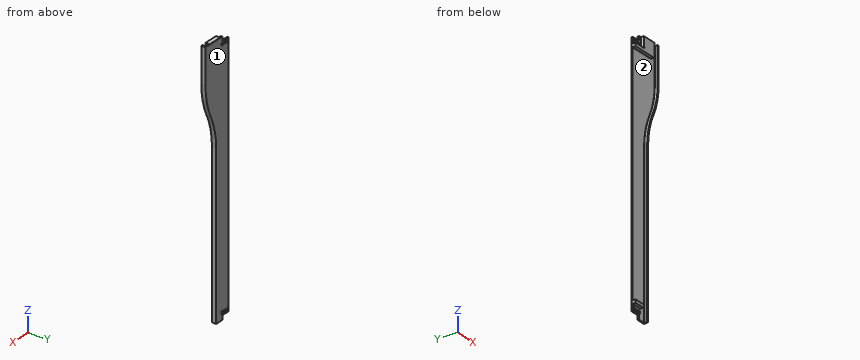
from build123d import *

# Parameters (mm, degrees)
EXTRUDE1_DEPTH                 = 10
EXTRUDE2_DEPTH                 = 7
SKETCH5_W                      = 20
SKETCH5_H                      = 15
SKETCH5_W_2                    = 26
EXTRUDE3_DEPTH                 = 7
SKETCH15_W                     = 6
SKETCH15_H                     = 10.7
SKETCH15_H_2                   = 25.7
EXTRUDE9_DEPTH                 = 7
F_8_CLEARANCE_HOLE1_AT_2_COUNT = 2
F_8_CLEARANCE_HOLE1_AT_2_PITCH = 15
EXTRUDE6_DEPTH                 = 4
SKETCH16_R                     = 1.5875
EXTRUDE10_DEPTH                = 7
CHAMFER1_SIZE                  = 0.3
CHAMFER2_SIZE                  = 0.5
CHAMFER3_SIZE                  = 0.3
FILLET3_R                      = 3
FILLET2_R                      = 0.5


with BuildPart() as part:
    # Sketch1 → Extrude1 (new body)
    with BuildSketch(Plane(origin=(0, 0, 0), x_dir=(1, 0, 0), z_dir=(0, 1, 0))):
        with BuildLine():
            Line((-93.1, 756.2), (-145.1, 756.2))
            Line((-145.1, 756.2), (-145.1, 766.9))
            Line((-145.1, 766.9), (-165.1, 766.9))
            Line((-165.1, 766.9), (-165.1, 1360.9))
            Line((-165.1, 1360.9), (-145.1, 1360.9))
            Line((-145.1, 1360.9), (-145.1, 1371.6))
            Line((-145.1, 1371.6), (-126.1, 1371.6))
            Line((-126.1, 1371.6), (-126.1, 990))
            ThreePointArc((-126.1, 990), (-121.926260039, 951.603222791), (-109.6, 915))
            ThreePointArc((-109.6, 915), (-97.273739961, 878.396777209), (-93.1, 840))
            Line((-93.1, 840), (-93.1, 756.2))
        make_face()
    extrude(amount=-EXTRUDE1_DEPTH)

    # Sketch4 → Extrude2 (cut)
    with BuildSketch(Plane.XZ.offset(10)):
        with BuildLine():
            Line((-165.1, -789.4), (-106.1, -789.4))
            Line((-106.1, -789.4), (-106.1, -756.2))
            Line((-106.1, -756.2), (-96.1, -756.2))
            Line((-96.1, -756.2), (-96.1, -840))
            ThreePointArc((-96.1, -840), (-100.203673361, -877.75219186), (-112.323006486, -913.740938573))
            ThreePointArc((-112.323006486, -913.740938573), (-124.856193439, -950.958637443), (-129.1, -990))
            Line((-129.1, -990), (-129.1, -1371.6))
            Line((-129.1, -1371.6), (-139.1, -1371.6))
            Line((-139.1, -1371.6), (-139.1, -1338.4))
            Line((-139.1, -1338.4), (-165.1, -1338.4))
            Line((-165.1, -1338.4), (-165.1, -789.4))
        make_face()
    extrude(amount=-EXTRUDE2_DEPTH, mode=Mode.SUBTRACT)

    # Sketch5 → Extrude3 (cut)
    with BuildSketch(Plane.XZ.offset(10)):
        with Locations((-155.1, -774.4)):
            Rectangle(SKETCH5_W, SKETCH5_H)
        with Locations((-152.1, -1353.4)):
            Rectangle(SKETCH5_W_2, SKETCH5_H)
    extrude(amount=-EXTRUDE3_DEPTH, mode=Mode.SUBTRACT)

    # Sketch15 → Extrude9 (cut)
    with BuildSketch(Plane.XZ.offset(10)):
        with Locations((-142.1, -1366.25)):
            Rectangle(SKETCH15_W, SKETCH15_H)
        with Locations((-142.1, -769.05)):
            Rectangle(SKETCH15_W, SKETCH15_H_2)
    extrude(amount=-EXTRUDE9_DEPTH, mode=Mode.SUBTRACT)

    # Sketch9 → 1/8 (0.125) Diameter Hole1 (revolve, cut)
    with BuildSketch(Plane(origin=(-152.6, -3, -772.9), x_dir=(0, 0, -1), z_dir=(1, 0, 0))):
        Polygon((0, 0), (0, 3), (2.2479, 3), (1.6129, 2.365), (1.6129, 0.635), (2.2479, 0), align=None)
    revolve(axis=Axis((-152.6, -9.35, -772.9), (0, 1, 0)), mode=Mode.SUBTRACT)

    # Sketch10 → #8 Clearance Hole1 (revolve, cut)
    with BuildSketch(Plane(origin=(-160.1, -3, -772.9), x_dir=(0, 0, -1), z_dir=(1, 0, 0))):
        Polygon((0, 0), (0, 3), (3.09245, 3), (2.45745, 2.365), (2.45745, 0.635), (3.09245, 0), align=None)
    f_8_clearance_hole1 = revolve(axis=Axis((-160.1, -9.35, -772.9), (0, 1, 0)), mode=Mode.SUBTRACT)

    # #8 Clearance Hole1 at 2: #8 Clearance Hole1 ×2
    with Locations(*[(i * F_8_CLEARANCE_HOLE1_AT_2_PITCH, 0, 0) for i in range(1, F_8_CLEARANCE_HOLE1_AT_2_COUNT)]):
        add(f_8_clearance_hole1, mode=Mode.SUBTRACT)

    # Sketch12 → Extrude6 (cut, through all)
    with BuildSketch(Plane.XZ.offset(3)):
        with BuildLine():
            Line((-154.251, -1353.9), (-154.251, -1355.9))
            ThreePointArc((-154.251, -1355.9), (-152.6, -1357.551), (-150.949, -1355.9))
            Line((-150.949, -1355.9), (-150.949, -1353.9))
            ThreePointArc((-150.949, -1353.9), (-152.6, -1352.249), (-154.251, -1353.9))
        make_face()
        with BuildLine():
            Line((-142.35, -1353.9), (-142.35, -1355.9))
            ThreePointArc((-142.35, -1355.9), (-145.1, -1358.65), (-147.85, -1355.9))
            Line((-147.85, -1355.9), (-147.85, -1353.9))
            ThreePointArc((-147.85, -1353.9), (-145.1, -1351.15), (-142.35, -1353.9))
        make_face()
        with BuildLine():
            Line((-162.85, -1353.9), (-162.85, -1355.9))
            ThreePointArc((-162.85, -1355.9), (-160.1, -1358.65), (-157.35, -1355.9))
            Line((-157.35, -1355.9), (-157.35, -1353.9))
            ThreePointArc((-157.35, -1353.9), (-160.1, -1351.15), (-162.85, -1353.9))
        make_face()
    extrude(amount=-EXTRUDE6_DEPTH, mode=Mode.SUBTRACT)

    # Sketch16 → Extrude10 (cut)
    with BuildSketch(Plane.XZ.offset(10)):
        with Locations((-139.1, -780.3125)):
            Circle(SKETCH16_R)
    extrude(amount=-EXTRUDE10_DEPTH, mode=Mode.SUBTRACT)

    # Chamfer1
    chamfer1_edges = [part.edges().sort_by_distance(p)[0] for p in [
        (-152.6, 0, -1352.249),
        (-150.949, 0, -1354.9),
        (-152.6, 0, -1357.551),
        (-154.251, 0, -1354.9),
        (-152.6, -3, -1352.249),
        (-154.251, -3, -1354.9),
        (-152.6, -3, -1357.551),
        (-150.949, -3, -1354.9),
    ]]
    chamfer(chamfer1_edges, length=CHAMFER1_SIZE)

    # Chamfer2
    chamfer2_edges = [part.edges().sort_by_distance(p)[0] for p in [
        (-94.6, -10, -756.2),
        (-93.1, -5, -756.2),
        (-119.1, 0, -756.2),
        (-145.1, -1.5, -756.2),
        (-106.1, -6.5, -756.2),
        (-101.1, -3, -756.2),
        (-96.1, -6.5, -756.2),
        (-126.1, -5, -1371.6),
        (-127.6, -10, -1371.6),
        (-129.1, -6.5, -1371.6),
        (-137.1, -3, -1371.6),
        (-145.1, -1.5, -1371.6),
        (-135.6, 0, -1371.6),
    ]]
    chamfer(chamfer2_edges, length=CHAMFER2_SIZE)

    # Chamfer3
    chamfer3_edges = [part.edges().sort_by_distance(p)[0] for p in [
        (-145.1, 0, -1351.15),
        (-142.35, 0, -1354.9),
        (-145.1, 0, -1358.65),
        (-147.85, 0, -1354.9),
        (-145.1, -3, -1351.15),
        (-147.85, -3, -1354.9),
        (-145.1, -3, -1358.65),
        (-142.35, -3, -1354.9),
        (-160.1, 0, -1351.15),
        (-157.35, 0, -1354.9),
        (-160.1, 0, -1358.65),
        (-162.85, 0, -1354.9),
        (-160.1, -3, -1351.15),
        (-162.85, -3, -1354.9),
        (-160.1, -3, -1358.65),
        (-157.35, -3, -1354.9),
    ]]
    chamfer(chamfer3_edges, length=CHAMFER3_SIZE)

    # Fillet3
    fillet3_edges = [part.edges().sort_by_distance(p)[0] for p in [
        (-106.1, -6.5, -789.4),
        (-139.1, -6.5, -1338.4),
        (-139.1, -6.5, -1345.9),
    ]]
    fillet(fillet3_edges, radius=FILLET3_R)

    # Fillet2
    fillet2_edges = [part.edges().sort_by_distance(p)[0] for p in [
        (-139.1, -3, -767.4625),
        (-137.5125, -3, -780.3125),
        (-96.1, -3, -798.35),
        (-139.1, -3, -1342.15),
        (-153.6, -3, -1338.4),
        (-106.1, -3, -771.55),
        (-139.978679656, -3, -1339.278679656),
        (-139.978679656, -3, -1345.021320344),
        (-106.978679656, -3, -788.521320344),
        (-137.1, -3, -789.4),
        (-100.203673361, -3, -877.75219186),
        (-124.856193439, -3, -950.958637443),
        (-129.1, -3, -1180.55),
        (-153.6, -3, -1345.9),
        (-152.1, -3, -781.9),
    ]]
    fillet(fillet2_edges, radius=FILLET2_R)


solid = part.part
The model under review builds one solid part; all positions refer to its coordinate system, in mm. Face numbers are marked on the shaded views. Give positions to 0.01 mm unless a question says otherwise; leave off trailing zeros. Order: outer loops, then holes, each group sorted by start corner. A loop starts at its lowest first (then second) coordinate and runs counter-clockwise, first axis right, second up. Notation, with made-up numbers: M 21.25,58 L 25.25,58 A15 ccw 25.25,81 Z; hole C 81,75 d6. An arc over 180 degrees is marked long. Use one line per item in the form item = value. Start each with the question number.
Item 1: The part is to be moulded in two halves that separate along Z. For the marked faces 1 and 2, say which applies: pulls with the +Z half, pulls with the -Z half, needs draft (parallel to the pull), parting line crosses it, or undercut.
Item 2: To check wall thickness, follow line 1 along X through (y, z) = (-1.15, -772.9); line 2 along Z through (x, y) = (-152.6, -1.55); line 3 along Z through (x, y) = (-160.1, -1.35). State the ranges of each line that lie inside material, in increasing order. Write a range as from..to.
Item 3: We need section A-A on z = -1143.5. Give the boundary of the cut face in (x, y), plus the area to 3 significant figures.
Item 4: Insertion check: pin 1 Ø5 at (x, y) = (-153.5, -7.5) entering from -Z; pin 2 Ø2.5 at (y, z) = (-1, -1364) entering from -X; pin 3 Ø0.6 at (y, z) = (-2, -1354.5) entering from +X; pin 4 Ø3 at (x, z) = (-160.1, -772.9) entering from +Y. Each pin has a flat end and moves straight along its axis. Give the tip position at first contact, or say it passes through.
Completed:
q1.face_1 = needs draft
q1.face_2 = undercut
q2.line_1 = -165.1..-162.56, -157.64..-154.21, -150.99..-147.56, -142.64..-93.1
q2.line_2 = -1360.9..-1357.55, -1352.25..-774.51, -771.29..-766.9
q2.line_3 = -1360.9..-1358.65, -1351.15..-775.36, -770.44..-766.9
q3.outline = M -165.1,-3 L -129.6,-3 A0.5 cw -129.1,-3.5 L -129.1,-10 L -126.1,-10 L -126.1,0 L -165.1,0 Z
q3.area = 138 mm²
q4.pin_1 = -1345.9
q4.pin_2 = -145.1
q4.pin_3 = -126.1
q4.pin_4 = through
